from build123d import *

# Parameters (mm, degrees)
F1_DEPTH = 52
F5_DEPTH = 25
F6_R     = 26
F7_R     = 25.99999


# Not quite as in the source:
# - a fillet or chamfer is up to 0.001 mm smaller than in the source, because OpenCascade refuses the exact size


with BuildPart() as f1:
    # F0 (on Top) → F1 (new body)
    with BuildSketch(Plane.XY):
        with BuildLine():
            Line((182, 38), (62.329768169, 38))
            ThreePointArc((62.329768169, 38), (-19.7348286497, 70.2818364741), (-73, 0))
            Line((-73, 0), (0, 0))
            Line((0, 0), (182, 0))
            Line((182, 0), (182, 38))
        make_face()
    extrude(amount=F1_DEPTH)

    # F2 (on face) → F3 (revolve, cut)
    with BuildSketch(Plane.XZ):
        Polygon((0, 52), (-60, 52), (-42, 0), (0, 0), align=None)
    revolve(axis=Axis((0, 0, 26), (0, 0, 1)), mode=Mode.SUBTRACT)

    # F4 (on face) → F5 (cut)
    with BuildSketch(Plane.XZ):
        with BuildLine():
            Line((87.3696654439, 26), (109.3696654439, 26))
            ThreePointArc((109.3696654439, 26), (98.3696654439, 37), (87.3696654439, 26))
        make_face()
        with BuildLine():
            ThreePointArc((157.3696654439, 26), (146.3696654439, 37), (135.3696654439, 26))
            Line((135.3696654439, 26), (157.3696654439, 26))
        make_face()
        with BuildLine():
            Line((157.3696654439, 26), (135.3696654439, 26))
            ThreePointArc((135.3696654439, 26), (146.3696654439, 15), (157.3696654439, 26))
        make_face()
        with BuildLine():
            ThreePointArc((87.3696654439, 26), (98.3696654439, 15), (109.3696654439, 26))
            Line((109.3696654439, 26), (87.3696654439, 26))
        make_face()
    extrude(amount=-F5_DEPTH, mode=Mode.SUBTRACT)

    # F6
    f6_edges = [f1.edges().sort_by_distance(p)[0] for p in [
        (182, 19, 52),
    ]]
    fillet(f6_edges, radius=F6_R)

    # F7 (radius 26 in the source; OpenCascade refuses exactly that, so slightly less here)
    f7_edges = [f1.edges().sort_by_distance(p)[0] for p in [
        (182, 19, 0),
    ]]
    fillet(f7_edges, radius=F7_R)


solid = f1.part
Geometry: final body of the model. Coordinates: model frame, mm. A direction names the side the tool comes from. Give positions to 0.01 mm unless a question says otherwise; leave off trailing zeros. Write each loop counter-clockwise with the first axis right and the second up, starting at its lowest first coordinate (ties: lowest second). Pieces come first, ordered by that corner, then holes. Notation, with made-up numbers: M 61.5,57.5 L 119.5,57.5 A11 ccw 119.5,74.5 Z; hole C -20.75,72 d10. An arc over 180 degrees is marked long. Answer in a Markdown table with one row per item. Add a question column.
(1) Ray query, line 1 (X direction, y = 3.5, z = 30.5); line 2 (X direction, y = 12.5, z = 30.5); line 3 (Y direction, x = 97, z = 18). Return the intervals inside material, ascending.
(2) Section A-A on z = 22.5. Return loops of the section in (x, y).
(3) Section B-B on x = 0. Return loops of the section in (y, z), and give its area (3 significant figures).
(4) Reachability of faces 1 (the flat face through (98, 25, 26)), 2 (the conical face through (1.075, 48.862, 19.858)) from +Z, -Z, +X, -X, +Y, -Y: full face, straight path, thin tool, end or side. Return the list, or none.
(5) First-contact query: pin 1 (3 mm diameter, centred on y = 52.5, z = 43.5, fed in from +X); pin 2 (3 mm diameter, centred on x = 139.5, z = 39.5, fed in from +Y); pin 3 (11 mm diameter, centred on x = 103, z = 30, fed in from -Y); pin 4 (4 mm diameter, centred on y = 52.5, z = 28.5, fed in from +X). Flat tips, straight axial feed; report the tip coordinate or a pass-through.
(6) Section C-C on y = 64.5. Return loops of the section in (x, z), and give its area (3 significant figures).
(7) Mould query, pull axis X, two halves, no side actions, for faces 3 (the cylindrical face through (-18.455, 70.629, 25.636)), 4 (the flat face through (146, 25, 26)), 5 (the flat face through (123, 38, 26)). Classes: +X half, -X half, draft (parallel to the pull), parting line (faces both ways), or undercut.
(8) Section D-D on z = 48. Return loops of the section in (x, y), and give its area (3 significant figures).
Result set:
| question | item | result |
|---|---|---|
| 1 | line 1 | x = -72.92 to -52.44, 52.44 to 88.33, 108.41 to 136.33, 156.41 to 181.61 |
| 1 | line 2 | x = -71.92 to -51.05, 51.05 to 88.33, 108.41 to 136.33, 156.41 to 181.61 |
| 1 | line 3 | y = 25 to 38 |
| 2 | outline | M -73,0 L -49.79,0 A49.79 cw 49.79,0 L 87.94,0 L 87.94,25 L 108.8,25 L 108.8,0 L 135.94,0 L 135.94,25 L 156.8,25 L 156.8,0 L 181.76,0 L 181.76,38 L 62.33,38 A73 ccw Z |
| 3 | outline | M 42,0 L 73,0 L 73,52 L 60,52 Z |
| 3 | area | 1,140 mm^2 |
| 4 | face 1 | -Y |
| 4 | face 2 | +Z, -Y |
| 5 | pin 1 | stops at x = 52.23 |
| 5 | pin 2 | stops at y = 38 |
| 5 | pin 3 | stops at y = 0 |
| 5 | pin 4 | stops at x = 52.71 |
| 6 | outline | M -34.19,0 L 34.19,0 L 34.19,52 L -34.19,52 Z |
| 6 | area | 3,560 mm^2 |
| 7 | face 3 | parting line |
| 7 | face 4 | undercut |
| 7 | face 5 | draft |
| 8 | outline | M -73,0 L -58.62,0 A58.62 cw 58.62,0 L 169.86,0 L 169.86,38 L 62.33,38 A73 ccw Z |
| 8 | area | 6,790 mm^2 |
